from build123d import *

# Parameters (mm, degrees)
DODANIE_WYCI_GNI_CIE1_DEPTH = 100
M5_CLEARANCE_HOLE1_D        = 5.5


with BuildPart() as part:
    # Szkic1 → Dodanie-wyciągnięcie1 (new body)
    with BuildSketch(Plane.XY):
        Polygon((0, 0), (0, 25), (25, 25), (25, 0), (23, 0), (23, 23), (2, 23), (2, 0), align=None)
    extrude(amount=DODANIE_WYCI_GNI_CIE1_DEPTH)

    # M5 Clearance Hole1 (through all)
    with Locations(Plane(origin=(0, 25, 0), x_dir=(1, 0, 0), z_dir=(0, 1, 0))):
        with Locations((13, -50), (13, -15), (13, -85)):
            Hole(M5_CLEARANCE_HOLE1_D / 2)


solid = part.part
Can you work these out from the model? Positions are in its coordinate system, mm. A direction names the side the tool comes from. Coordinates: 2 decimals unless noted, no trailing zeros. Write each loop counter-clockwise with the first axis right and the second up, starting at its lowest first coordinate (ties: lowest second). Pieces come first, ordered by that corner, then holes. Notation, with made-up numbers: M -12,-29.75 L 35,-29.75 A18 ccw 35,-14.75 Z; hole C 63,35 d7. An arc over 180 degrees is marked long. Use one line per item in the form item = value.
Q1. For faces 1 (the flat face through (10, 23, 49)), 2 (the cylindrical face through (13.358, 23.986, 12.273)), which set-ups out of +Z, -Z, +X, -X, +Y, -Y let a thin tool reach every point of the face, with its end or its side?
Model answer:
face_1 = +Z, -Z, -Y
face_2 = +Y, -Y
Q2. For P1, Ø8, axis at x = 13.5, z = 47.5, coming from the -Y side; P2, Ø7, axis at x = 13, z = 85, coming from the +Y side; P3, Ø5, axis at x = 13, z = 50, coming from the +Y side, each with a flat end and sliding along its axis, tell me the tip position at first contact or that it passes through.
Model answer:
P1 = 23
P2 = 25
P3 = through
Q3. If we section it at A-A (x = 13): Write out the boundary of the cut face in (y, z), then the cut area to 3 significant figures.
Model answer:
outline = M 23,0 L 25,0 L 25,12.25 L 23,12.25 Z; M 23,17.75 L 25,17.75 L 25,47.25 L 23,47.25 Z; M 23,52.75 L 25,52.75 L 25,82.25 L 23,82.25 Z; M 23,87.75 L 25,87.75 L 25,100 L 23,100 Z
area = 167 mm^2
Q4. If we section it at D-D (z = 42): Write out the boundary of the cut face in (x, y), then the cut area to 3 significant figures.
Model answer:
outline = M 0,0 L 2,0 L 2,23 L 23,23 L 23,0 L 25,0 L 25,25 L 0,25 Z
area = 142 mm^2
Q5. If we section it at C-C (y = 15.25): Write out the boundary of the cut face in (x, z), then the cut area to 3 significant figures.
Model answer:
outline = M 0,0 L 2,0 L 2,100 L 0,100 Z; M 23,0 L 25,0 L 25,100 L 23,100 Z
area = 400 mm^2
Q6. I need wall thicknesses on line 1 along Z through (x, y) = (13, 24.5); line 2 along X through (y, z) = (3.25, 57); line 3 along X through (y, z) = (24.4, 50). Which ranges of each line are inside material? Lowest first, please. Write a range as from..to.
Model answer:
line_1 = 0..12.25, 17.75..47.25, 52.75..82.25, 87.75..100
line_2 = 0..2, 23..25
line_3 = 0..10.25, 15.75..25
Q7. If we section it at B-B (z = 85): Write out the boundary of the cut face in (x, y), then the cut area to 3 significant figures.
Model answer:
outline = M 0,0 L 2,0 L 2,23 L 10.25,23 L 10.25,25 L 0,25 Z; M 15.75,23 L 23,23 L 23,0 L 25,0 L 25,25 L 15.75,25 Z
area = 131 mm^2
Q8. We'd pull the mould along X, two halves only. Please class faces 3 (the flat face through (2, 12, 49)), 4 (the flat face through (0, 12, 49)), 5 (the flat face through (1, 0, 49)): +X half, -X half, draft (parallel to the pull), parting line (faces both ways), or undercut.
Model answer:
face_3 = undercut
face_4 = -X half
face_5 = draft
